```python
from build123d import *


with BuildPart() as part:
    # Szkic1 → Obrót1 (revolve)
    with BuildSketch(Plane.XY, mode=Mode.PRIVATE) as obr_t1_sk:
        with BuildLine():
            Line((-30.5, 15.342508556), (-42, 15.342508556))
            Line((-42, 15.342508556), (-42, 11.842508556))
            Line((-42, 11.842508556), (-39.351466792, 11.842508556))
            ThreePointArc((-39.351466792, 11.842508556), (-39.253071436, 11.760351037), (-39.316354447, 11.648875638))
            Line((-39.316354447, 11.648875638), (-42, 10.642508556))
            Line((-42, 10.642508556), (-42, 10.342508556))
            Line((-42, 10.342508556), (-37, 10.842508556))
            Line((-37, 10.842508556), (-30.5, 10.342508556))
            Line((-30.5, 10.342508556), (-30.5, 10.642508556))
            Line((-30.5, 10.642508556), (-35.639658009, 11.986726805))
            ThreePointArc((-35.639658009, 11.986726805), (-35.938355792, 12.365172989), (-35.656081251, 12.756022017))
            Line((-35.656081251, 12.756022017), (-30.5, 14.342508556))
            Line((-30.5, 14.342508556), (-30.5, 15.342508556))
        make_face()
    revolve(obr_t1_sk.sketch.rotate(Axis((-61.483966901, 0.342508556, 0), (1, 0, 0)), 90), axis=Axis((-61.483966901, 0.342508556, 0), (1, 0, 0)))


solid = part.part
```
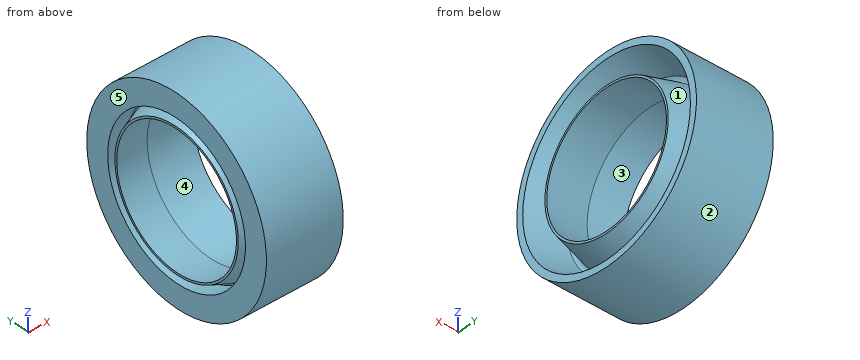
Source: CAD feature listing. Evaluate the final solid. Frame: model axes, mm. Face numbers are marked on the shaded views. A direction names the side the tool comes from. Give positions to 0.01 mm unless a question says otherwise; leave off trailing zeros. Loops run counter-clockwise (first coordinate to the right, second up) from the corner with the lowest first, then second, coordinate; pieces in that order, holes last. Notation, with made-up numbers: M 67.5,58 L 122.5,58 A26 cw 122.5,90 Z; hole C -5.75,61 d5. An arc over 180 degrees is marked long. Put each result on its own line as item: value.
Q1. Reachability of the marked faces 4 and 5 from +Z, -Z, +X, -X, +Y, -Y: full face, straight path, thin tool, end or side. Return the list, or none.
Response values:
face 4: none
face 5: +Z, -Z, -X, +Y, -Y
Q2. Section C-C (x = -32.75). Return the cut outline in (y, z).
Response values:
outline: C 0.34,0 d30; C 0.34,0 d21.78; hole C 0.34,0 d26.62; hole C 0.34,0 d20.35
Q3. Line query: probe 1 along Y at (x, z) = (-33.5, -6); probe 2 along Z at (x, y) = (-32.25, -1.75); probe 3 along Y at (x, z) = (-35.5, -4.5). Output: solid intervals per line, ascending. Write a range as [from, to].
Response values:
probe 1: y = [-13.41, -11.28], [-8.98, -7.94], [8.63, 9.66], [11.96, 14.09]
probe 2: z = [-14.85, -13.3], [-10.55, -9.92], [9.92, 10.55], [13.3, 14.85]
probe 3: y = [-13.97, -11.28], [-10.36, -9.02], [9.7, 11.04], [11.96, 14.65]
Q4. Section A-A (z = 0). Return the cut outline in (x, y), and give its area (3 significant figures).
Response values:
outline: M -42,-14.66 L -30.5,-14.66 L -30.5,-13.66 L -35.66,-12.07 A0.4 cw -35.64,-11.3 L -30.5,-9.96 L -30.5,-9.66 L -37,-10.16 L -42,-9.66 L -42,-9.96 L -39.32,-10.96 A0.1 cw -39.35,-11.16 L -42,-11.16 Z; M -42,10.34 L -37,10.84 L -30.5,10.34 L -30.5,10.64 L -35.64,11.99 A0.4 cw -35.66,12.76 L -30.5,14.34 L -30.5,15.34 L -42,15.34 L -42,11.84 L -39.35,11.84 A0.1 cw -39.32,11.65 L -42,10.64 Z
area: 82.2 mm²
Q5. Section B-B (x = -34.75). Return the cut outline in (y, z).
Response values:
outline: C 0.34,0 d30; C 0.34,0 d22.82; hole C 0.34,0 d25.38; hole C 0.34,0 d20.65
Q6. Pin query (flat end, axial travel): P1, Ø2, axis at x = -37, y = 4.5, coming from the -Z side; P2, Ø3, axis at x = -33, z = -2, coming from the +Y side; P3, Ø5, axis at x = -34.5, z = 10, coming from the +Y side. Return the tip coordinate at first contact, or that it passes through.
Response values:
P1: stops at z = -14.66
P2: stops at y = 15.33
P3: stops at y = 13.33
Q7. Mould query, pull axis X, two halves, no side actions, for the marked faces 1, 2 and 3. Classes: released by +X, released by -X, zero draft, split by the parting line, or undercut.
Response values:
face 1: released by +X
face 2: zero draft
face 3: undercut
